Verification items for the finished model (mm, model axes). Face numbers are marked on the shaded views. A direction names the side the tool comes from. Round coordinates to 2 decimals unless told otherwise and drop trailing zeros. Loops run counter-clockwise (first coordinate to the right, second up) from the corner with the lowest first, then second, coordinate; pieces in that order, holes last. Notation, with made-up numbers: (79, 22.5) -> (83, 22.5) arc R18 ccw to (83, 45.5) -> close; hole circle Ø10 at (87, -34). An arc over 180 degrees is marked (long way). Use a Markdown table: item, result. Add a question column.
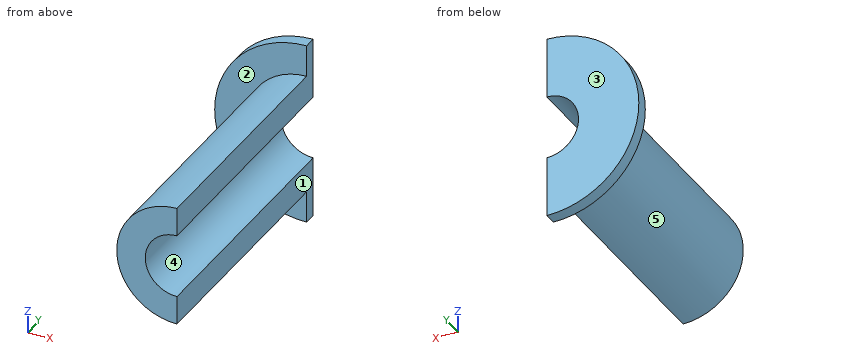
```python
from build123d import *

# Parameters (mm, degrees)
F2_R     = 6.35
F3_DEPTH = 101.6
F5_DEPTH = 127


with BuildPart() as f1:
    # F0 (on Top) → F1 (revolve)
    with BuildSketch(Plane.XY):
        Polygon((0, 37.726658), (0, -15.613342), (12.065, -15.613342), (12.065, 35.186658), (18.415, 35.186658), (18.415, 37.726658), align=None)
    revolve(axis=Axis((0, 11.056658, 0), (0, -1, 0)))

    # F2 (on face) → F3 (cut)
    with BuildSketch(Plane(origin=(0, 37.726658, 0), x_dir=(-1, 0, 0), z_dir=(0, 1, 0))):
        Circle(F2_R)
    extrude(amount=-F3_DEPTH, mode=Mode.SUBTRACT)

    # F4 (on face) → F5 (cut)
    with BuildSketch(Plane(origin=(0, 37.726658, 0), x_dir=(-1, 0, 0), z_dir=(0, 1, 0))):
        Polygon((0, 18.415), (0, 18.85934), (0, 32.270402), (-18.049083, 25.601261), (-23.923116, -16.779846), (0, -20.095596), align=None)
    extrude(amount=-F5_DEPTH, mode=Mode.SUBTRACT)


solid = f1.part
```
1) Go/stop test with flat-tipped pins: pin 1 (1.5 mm diameter, centred on y = 16, z = 10, fed in from -X); pin 2 (4 mm diameter, centred on x = -11.5, y = -10, fed in from +Z); pin 3 (12 mm diameter, centred on y = 7, z = 10, fed in from -X). Record where each tip stops, or that it passes through.
2) Access from +Z, -Z, +X, -X, +Y, -Y to the whole of each face (thin tool, end or side, straight path). Record for the marked faces 1 and 2.
3) Sectioned sample at A-A on x = -10.5. Enter the section's corners in (y, z), then the cut area to 3 significant figures.
4) Release check for a two-part mould opening along Z. For the marked faces 3, 4 and 5 record: released by +Z, released by -Z, zero draft, split by the parting line, or undercut.
5) Sectioned sample at B-B on z = 0. Enter the section's corners in (x, y) (3 decimals).
6) Thickness scan on line 1 (Y direction, x = -13.5, z = -3); line 2 (Z direction, x = -4.25, y = 20.5); line 3 (Z direction, x = -2.5, y = -9). Record the ranges inside material, lowest first.
7) Sectioned sample at C-C on y = 12. Enter the section's corners in (x, z) (3 decimals).
Geometry results:
| question | item | result |
|---|---|---|
| 1 | pin 1 | x = -7.75 |
| 1 | pin 2 | z = 7.44 |
| 1 | pin 3 | x = -11.38 |
| 2 | face 1 | +Z, -Z, +X, +Y, -Y |
| 2 | face 2 | -X, -Y |
| 3 | outline | (-15.61, -5.94) -> (35.19, -5.94) -> (35.19, -15.13) -> (37.73, -15.13) -> (37.73, 15.13) -> (35.19, 15.13) -> (35.19, 5.94) -> (-15.61, 5.94) -> close |
| 3 | area | 681 mm^2 |
| 4 | face 3 | zero draft |
| 4 | face 4 | undercut |
| 4 | face 5 | split by the parting line |
| 5 | outline | (-18.415, 35.187) -> (-12.065, 35.187) -> (-12.065, -15.613) -> (-6.35, -15.613) -> (-6.35, 37.727) -> (-18.415, 37.727) -> close |
| 6 | line 1 | 35.19 to 37.73 |
| 6 | line 2 | -11.29 to -4.72, 4.72 to 11.29 |
| 6 | line 3 | -11.8 to -5.84, 5.84 to 11.8 |
| 7 | outline | (0, -12.065) -> (0, -6.35) arc R6.35 cw to (0, 6.35) -> (0, 12.065) arc R12.065 ccw to start |
